```python
from build123d import *

# Parameters (mm, degrees)
F0_R     = 6
F1_DEPTH = 4
F0_R_2   = 4
F2_DEPTH = 3


with BuildPart() as f1:
    # F0 (on Right) → F1 (new body, symmetric)
    with BuildSketch(Plane.YZ):
        with BuildLine():
            ThreePointArc((-5.4605056446, 10.6856388721), (-6.2639417408, -10.2353814715), (12, 0))
            ThreePointArc((12, 0), (10.2353814715, 6.2639417408), (5.4605056446, 10.6856388721))
            ThreePointArc((5.4605056446, 10.6856388721), (0, 12), (-5.4605056446, 10.6856388721))
        make_face()
        Circle(F0_R, mode=Mode.SUBTRACT)
    extrude(amount=F1_DEPTH, both=True)



with BuildPart() as f1b:
    # F0 (on Right) → F1, piece 2 (new body, symmetric)
    with BuildSketch(Plane.YZ):
        with BuildLine():
            ThreePointArc((-5.4605056446, 44.1533874675), (0, 42), (5.4605056446, 44.1533874675))
            ThreePointArc((5.4605056446, 44.1533874675), (7.3377123532, 46.8128417953), (8, 50))
            ThreePointArc((8, 50), (-3.1871582047, 57.3377123532), (-5.4605056446, 44.1533874675))
        make_face()
        with Locations((0, 50)):
            Circle(F0_R_2, mode=Mode.SUBTRACT)
    extrude(amount=F1_DEPTH, both=True)


with BuildPart() as f1_1:
    add(f1.part)

    add(f1b.part)  # F2 merges F1b
    # F0 (on Right) → F2 (join, symmetric)
    with BuildSketch(Plane.YZ):
        with BuildLine():
            ThreePointArc((-5.4605056446, 10.6856388721), (0, 12), (5.4605056446, 10.6856388721))
            Line((5.4605056446, 10.6856388721), (5.4605056446, 44.1533874675))
            ThreePointArc((5.4605056446, 44.1533874675), (0, 42), (-5.4605056446, 44.1533874675))
            Line((-5.4605056446, 44.1533874675), (-5.4605056446, 10.6856388721))
        make_face()
    extrude(amount=F2_DEPTH, both=True)


solid = f1_1.part
```
Geometry check sheet. Reference: the model listing, model coordinates, mm. A direction names the side the tool comes from. Give positions to 0.01 mm unless a question says otherwise; leave off trailing zeros. Write each loop counter-clockwise with the first axis right and the second up, starting at its lowest first coordinate (ties: lowest second). Pieces come first, ordered by that corner, then holes. Notation, with made-up numbers: (53.25, -28.75) - (91.25, -28.75) arc R24 cw to (91.25, 4.25) - close; hole circle Ø8 at (-24.5, 21). An arc over 180 degrees is marked (long way). Use a Markdown table: item, result.
Q1. Thickness scan on L1, parallel to Z at x = -1.8, y = 0; L2, parallel to Z at x = -1, y = 1; L3, parallel to X at y = -2, z = 39.5. Record the ranges inside material, lowest first. Write a range as [from, to].
Computed:
| item | result |
|---|---|
| L1 | z = [-12, -6], [6, 46], [54, 58] |
| L2 | z = [-11.96, -5.92], [5.92, 46.13], [53.87, 57.94] |
| L3 | x = [-3, 3] |
Q2. Set-up check for faces 1 (the face through (0, 5.461, 27)), 2 (the face through (-4, -6, -2)): record each of +Z, -Z, +X, -X, +Y, -Y from which the full face is reachable in a straight line by a thin tool's end or side.
Computed:
| item | result |
|---|---|
| face 1 | +X, -X, +Y |
| face 2 | +Z, -Z, -X, +Y, -Y |
Q3. Section check C-C, the plane y = 2.75. Enter the section's corners in (x, z).
Computed:
| item | result |
|---|---|
| outline | (-4, -11.68) - (4, -11.68) - (4, -5.33) - (-4, -5.33) - close; (-4, 5.33) - (4, 5.33) - (4, 11.68) - (3, 11.68) - (3, 42.49) - (4, 42.49) - (4, 47.1) - (-4, 47.1) - (-4, 42.49) - (-3, 42.49) - (-3, 11.68) - (-4, 11.68) - close; (-4, 52.9) - (4, 52.9) - (4, 57.51) - (-4, 57.51) - close |
Q4. Section check A-A, the plane y = 0. Enter the section's corners in (x, z).
Computed:
| item | result |
|---|---|
| outline | (-4, -12) - (4, -12) - (4, -6) - (-4, -6) - close; (-4, 6) - (4, 6) - (4, 12) - (3, 12) - (3, 42) - (4, 42) - (4, 46) - (-4, 46) - (-4, 42) - (-3, 42) - (-3, 12) - (-4, 12) - close; (-4, 54) - (4, 54) - (4, 58) - (-4, 58) - close |
Q5. Section check B-B, the plane x = 1. Enter the section's corners in (y, z), then the cut area to 3 significant figures.
Computed:
| item | result |
|---|---|
| outline | (-5.46, 10.69) arc R12 ccw (long way) to (5.46, 10.69) - (5.46, 44.15) arc R8 ccw (long way) to (-5.46, 44.15) - close; hole circle Ø12 at (0, 0); hole circle Ø8 at (0, 50) |
| area | 830 mm² |
Q6. Go/stop test with flat-tipped pins: P1, Ø1, axis at x = 0, y = 9, coming from the -Z side; P2, Ø1, axis at x = 1.5, y = -7, coming from the +Z side; P3, Ø10.5, axis at y = 0, z = 50, coming from the +X side; P4, Ø1.5, axis at x = -2, z = 6, coming from the +Y side. Record where each tip stops, or that it passes through.
Computed:
| item | result |
|---|---|
| P1 | stops at z = -8.47 |
| P2 | stops at z = 54.66 |
| P3 | stops at x = 4 |
| P4 | stops at y = 10.79 |
Q7. Draft check along Z on faces 3 (the face through (0, -5.461, 28)), 4 (the face through (4, -6, -2)). Enter one of: pulls with the +Z half, pulls with the -Z half, needs draft (parallel to the pull), parting line crosses it, or undercut.
Computed:
| item | result |
|---|---|
| face 3 | undercut |
| face 4 | needs draft |
Q8. Section check D-D, the plane z = 30.5. Enter the section's corners in (x, y), then the cut area to 3 significant figures.
Computed:
| item | result |
|---|---|
| outline | (-3, -5.46) - (3, -5.46) - (3, 5.46) - (-3, 5.46) - close |
| area | 65.5 mm² |
